Autodesk Inventor part; units mm, degrees
ref_plane "YZ Plane" through (0, 0, 0) normal (1, 0, 0) x (0, 1, 0)
ref_plane "XZ Plane" through (0, 0, 0) normal (0, 1, 0) x (-1, 0, 0)
ref_plane "XY Plane" through (0, 0, 0) normal (0, 0, 1) x (1, 0, 0)
sketch "スケッチ1" plane through (0, 0, 0) normal (0, 0, 1) x (1, 0, 0)
  circle A0 centre (37, 36) radius 2.75
  line L0 (42, 30.5) -> (42, 41.5)
  line L1 (28, 41.5) -> (42, 41.5)
  line L2 (28, 30.5) -> (28, 41.5)
  line L3 (42, 30.5) -> (28, 30.5)
  circle A1 centre (5, 36) radius 2.75
  line L4 (14, 30.5) -> (14, 41.5)
  line L5 (0, 41.5) -> (14, 41.5)
  line L6 (0, 30.5) -> (0, 41.5)
  line L7 (14, 30.5) -> (0, 30.5)
  circle A2 centre (37, 0) radius 2.75
  line L8 (42, -5.5) -> (42, 5.5)
  line L9 (28, 5.5) -> (42, 5.5)
  line L10 (28, -5.5) -> (28, 5.5)
  line L11 (42, -5.5) -> (28, -5.5)
  circle A3 centre (5, 0) radius 2.75
  line L12 (14, -5.5) -> (14, 5.5)
  line L13 (0, 5.5) -> (14, 5.5)
  line L14 (0, -5.5) -> (0, 5.5)
  line L15 (14, -5.5) -> (0, -5.5)
  line L16 (0, -5.5) -> (42, -5.5)
  line L17 (42, -5.5) -> (42, 41.5)
  line L18 (42, 41.5) -> (0, 41.5)
  line L19 (0, 41.5) -> (0, -5.5)
  point P0 (0, 0)
extrude "押し出し1" add sketch "スケッチ1" along normal blind 10
sketch "スケッチ2" plane through (0, 0, 10) normal (0, 0, 1) x (1, 0, 0)
  circle A0 centre (18.766, 18.4051) radius 10
  point P0 (0, 0)
  dimension "d2" = 20
extrude "押し出し2" add sketch "スケッチ2" along normal blind 160
CAD build for the part. Positions are in the model's coordinates, mm. Round coordinates to 2 decimals unless told otherwise and drop trailing zeros. Loops run counter-clockwise (first coordinate to the right, second up) from the corner with the lowest first, then second, coordinate; pieces in that order, holes last. Notation, with made-up numbers: M 72,49 L 130,49 A12 cw 130,62 Z; hole C 37.25,38.25 d7. An arc over 180 degrees is marked long. Use a Markdown table: item, result. Add a question column.
(1) Cut at D-D (y = 24.5). Give the cut face in (x, z).
(2) Drill centre lines: line 1 (Y direction, x = 37, z = 3); line 2 (Z direction, x = 34, y = 2.5); line 3 (Y direction, x = 19.5, z = 113). Where is each one in solid material? Low to high.
(3) Flat gauge pins, fed straight in: pin 1 (1 mm diameter, centred on y = 25, z = 123, fed in from +X); pin 2 (4 mm diameter, centred on x = 31, z = 104.5, fed in from -Y); pin 3 (4 mm diameter, centred on y = 24, z = 21, fed in from -X); pin 4 (6 mm diameter, centred on y = 27.5, z = 73, fed in from -X). Where does each tip first touch, or does it go through?
(4) Pull direction Y, two halves, no side cores. Call faces 1 (the face through (28.304, 15.401, 88.88)), 2 (the face through (4.642, 33.273, 4.93)), 3 (the face through (0, 18, 5)), 4 (the face through (21, -5.5, 5)): +Y half, -Y half, draft (parallel to the pull), parting line (faces both ways), or undercut.
(5) Cut at B-B (y = 0). Give the cut face in (x, z).
(6) Cut at A-A (x = 37). Give the cut face in (y, z), and give its area (3 significant figures).
(7) Cut at C-C (x = 26). Give the cut face in (y, z).
Geometry says:
| question | item | result |
|---|---|---|
| 1 | outline | M 0,0 L 42,0 L 42,10 L 26.69,10 L 26.69,170 L 10.84,170 L 10.84,10 L 0,10 Z |
| 2 | line 1 | y = -5.5 to -2.75, 2.75 to 33.25, 38.75 to 41.5 |
| 2 | line 2 | z = 0 to 10 |
| 2 | line 3 | y = 8.43 to 28.38 |
| 3 | pin 1 | stops at x = 26.69 |
| 3 | pin 2 | passes through |
| 3 | pin 3 | stops at x = 9.43 |
| 3 | pin 4 | stops at x = 10.84 |
| 4 | face 1 | parting line |
| 4 | face 2 | undercut |
| 4 | face 3 | draft |
| 4 | face 4 | -Y half |
| 5 | outline | M 0,0 L 2.25,0 L 2.25,10 L 0,10 Z; M 7.75,0 L 34.25,0 L 34.25,10 L 7.75,10 Z; M 39.75,0 L 42,0 L 42,10 L 39.75,10 Z |
| 6 | outline | M -5.5,0 L -2.75,0 L -2.75,10 L -5.5,10 Z; M 2.75,0 L 33.25,0 L 33.25,10 L 2.75,10 Z; M 38.75,0 L 41.5,0 L 41.5,10 L 38.75,10 Z |
| 6 | area | 360 mm² |
| 7 | outline | M -5.5,0 L 41.5,0 L 41.5,10 L 25.31,10 L 25.31,170 L 11.5,170 L 11.5,10 L -5.5,10 Z |
